```python
from build123d import *

# Parameters (mm, degrees)
F0_R     = 7.9375
F1_DEPTH = 3.175


with BuildPart() as f1:
    # F0 (on Top) → F1 (new body)
    with BuildSketch(Plane.XY):
        with BuildLine():
            Line((-43.533407, 61.9125), (-80.9625, 61.9125))
            ThreePointArc((-80.9625, 61.9125), (-88.505359, 59.759164), (-93.774579, 53.948235))
            ThreePointArc((-93.774579, 53.948235), (-106.3625, 0), (-93.774579, -53.948235))
            ThreePointArc((-93.774579, -53.948235), (-88.505359, -59.759164), (-80.9625, -61.9125))
            Line((-80.9625, -61.9125), (-43.533407, -61.9125))
            ThreePointArc((-43.533407, -61.9125), (-41.755051, -62.166604), (-40.119022, -62.908578))
            ThreePointArc((-40.119022, -62.908578), (-29.365201, -68.59089), (-17.831054, -72.450526))
            ThreePointArc((-17.831054, -72.450526), (-15.121491, -73.877949), (-13.395178, -76.407596))
            ThreePointArc((-13.395178, -76.407596), (0, -85.725), (13.395178, -76.407596))
            ThreePointArc((13.395178, -76.407596), (15.121491, -73.877949), (17.831054, -72.450526))
            ThreePointArc((17.831054, -72.450526), (29.365201, -68.59089), (40.119022, -62.908578))
            ThreePointArc((40.119022, -62.908578), (41.755051, -62.166604), (43.533407, -61.9125))
            Line((43.533407, -61.9125), (80.9625, -61.9125))
            ThreePointArc((80.9625, -61.9125), (88.505359, -59.759164), (93.774579, -53.948235))
            ThreePointArc((93.774579, -53.948235), (106.3625, 0), (93.774579, 53.948235))
            ThreePointArc((93.774579, 53.948235), (88.505359, 59.759164), (80.9625, 61.9125))
            Line((80.9625, 61.9125), (43.533407, 61.9125))
            ThreePointArc((43.533407, 61.9125), (41.755051, 62.166604), (40.119022, 62.908578))
            ThreePointArc((40.119022, 62.908578), (29.365201, 68.59089), (17.831054, 72.450526))
            ThreePointArc((17.831054, 72.450526), (15.121491, 73.877949), (13.395178, 76.407596))
            ThreePointArc((13.395178, 76.407596), (0, 85.725), (-13.395178, 76.407596))
            ThreePointArc((-13.395178, 76.407596), (-15.121491, 73.877949), (-17.831054, 72.450526))
            ThreePointArc((-17.831054, 72.450526), (-29.365201, 68.59089), (-40.119022, 62.908578))
            ThreePointArc((-40.119022, 62.908578), (-41.755051, 62.166604), (-43.533407, 61.9125))
        make_face()
        with Locations((-80.9625, -47.625)):
            Circle(F0_R, mode=Mode.SUBTRACT)
        with Locations((0, -71.4375)):
            Circle(F0_R, mode=Mode.SUBTRACT)
        with Locations((80.9625, -47.625)):
            Circle(F0_R, mode=Mode.SUBTRACT)
        with Locations((-80.9625, 47.625)):
            Circle(F0_R, mode=Mode.SUBTRACT)
        with BuildLine():
            ThreePointArc((26.800085, -41.275), (0, -49.2125), (-26.800085, -41.275))
            Line((-26.800085, -41.275), (-49.2125, -41.275))
            ThreePointArc((-49.2125, -41.275), (-90.4875, 0), (-49.2125, 41.275))
            Line((-49.2125, 41.275), (-26.800085, 41.275))
            ThreePointArc((-26.800085, 41.275), (0, 49.2125), (26.800085, 41.275))
            Line((26.800085, 41.275), (49.2125, 41.275))
            ThreePointArc((49.2125, 41.275), (90.4875, 0), (49.2125, -41.275))
            Line((49.2125, -41.275), (26.800085, -41.275))
        make_face(mode=Mode.SUBTRACT)
        with Locations((0, 71.4375)):
            Circle(F0_R, mode=Mode.SUBTRACT)
        with Locations((80.9625, 47.625)):
            Circle(F0_R, mode=Mode.SUBTRACT)
    extrude(amount=F1_DEPTH)


solid = f1.part
```
Can you work these out from the model? Positions are in its coordinate system, mm. A direction names the side the tool comes from. Round coordinates to 2 decimals unless told otherwise and drop trailing zeros. Loops run counter-clockwise (first coordinate to the right, second up) from the corner with the lowest first, then second, coordinate; pieces in that order, holes last.
Item 1: Suppose I cut it at D-D, the plane z = 1.3. State how many separate pieces and enclosed holes the cut face has, then the cut area to 3 significant figures.
Item 2: Please list where these lines run through material, in increasing order: L1, parallel to X at y = 1, z = 1.2; L2, parallel to Y at x = 79, z = 1.75; L3, parallel to X at y = 53.5, z = 1.
Item 3: Suppose I cut it at C-C, the plane x = -70.5. Write out the boundary of the cut face in (y, z) (1 decimal).
Item 4: Suppose I cut it at B-B, the plane y = 0. Write out the boundary of the cut face in (x, z) (1 decimal), then the cut area to 3 significant figures.
Item 5: Suppose I cut it at A-A, the plane x = 0. Write out the boundary of the cut face in (y, z) (1 decimal).
Item 6: Which directions (+Z, -Z, +X, -X, +Y, -Y) give clear straight access to the entire face, cutting with the end or side of a thin tool? Please do faces 4 (the cylindrical face through (-90.478, -0.908, 1.565)), 5 (the flat face through (23, 45, 0)).
Item 7: If we mould it in two halves opening along Y, with no side actions, what happens to faces 1 (the cylindrical face through (90.478, 0.908, 1.565)), 2 (the cylindrical face through (-29.522, -68.524, 1.565)), 3 (the cylindrical face through (-88.41, 59.82, 1.57))? For each: +Y half, -Y half, draft (parallel to the pull), parting line (faces both ways), or undercut.
Item 8: Will these pins go through, and if not, where does the flat tip stop? pin 1 Ø1 at (x, z) = (42.5, 1) entering from -Y; pin 2 Ø1 at (x, z) = (24.5, 0.5) entering from +Y; pin 3 Ø1 at (x, z) = (42.5, 1) entering from +Y; pin 4 Ø12.5 at (x, y) = (80.96, 47.62) entering from -Z.
Reported:
1. separate pieces: 1
1. enclosed holes: 7
1. area: 11,600 mm2
2. L1: x = -106.36 to -90.48, 90.48 to 106.36
2. L2: y = -61.91 to -55.32, -39.93 to -28.57, 28.57 to 39.93, 55.32 to 61.91
2. L3: x = -93.99 to -86.3, -75.63 to 75.63, 86.3 to 93.99
3. outline: (-61.9, 0) - (-35.4, 0) - (-35.4, 3.2) - (-61.9, 3.2) - close; (35.4, 0) - (61.9, 0) - (61.9, 3.2) - (35.4, 3.2) - close
4. outline: (-106.4, 0) - (-90.5, 0) - (-90.5, 3.2) - (-106.4, 3.2) - close; (90.5, 0) - (106.4, 0) - (106.4, 3.2) - (90.5, 3.2) - close
4. area: 101 mm2
5. outline: (-85.7, 0) - (-79.4, 0) - (-79.4, 3.2) - (-85.7, 3.2) - close; (-63.5, 0) - (-49.2, 0) - (-49.2, 3.2) - (-63.5, 3.2) - close; (49.2, 0) - (63.5, 0) - (63.5, 3.2) - (49.2, 3.2) - close; (79.4, 0) - (85.7, 0) - (85.7, 3.2) - (79.4, 3.2) - close
6. face 4: +Z, -Z
6. face 5: -Z, +X, -X, +Y, -Y
7. face 1: undercut
7. face 2: -Y half
7. face 3: +Y half
8. pin 1: stops at y = -62.1
8. pin 2: stops at y = 70.65
8. pin 3: stops at y = 62.1
8. pin 4: passes through
